```python
from build123d import *

# Parameters (mm, degrees)
BOSS_EXTRUDE1_DEPTH = 7.5
SKETCH3_W           = 56.5
SKETCH3_H           = 84.5
SKETCH3_W_2         = 54.5
SKETCH3_H_2         = 69.44
CUT_EXTRUDE1_DEPTH  = 5
SKETCH4_W           = 54.5
SKETCH4_H           = 9.636528607
CUT_EXTRUDE2_DEPTH  = 5
SKETCH5_W           = 32
SKETCH5_H           = 23.1
BOSS_EXTRUDE2_DEPTH = 49
SKETCH6_W           = 32
SKETCH6_H           = 23.1
BOSS_EXTRUDE3_DEPTH = 49
SKETCH7_R           = 5.000174567
BOSS_EXTRUDE4_DEPTH = 20


with BuildPart() as part:
    # Sketch2 → Boss-Extrude1 (new body)
    with BuildSketch(Plane.XY):
        with BuildLine():
            Line((-82.896774194, 76.290322581), (37.103225806, 76.290322581))
            ThreePointArc((37.103225806, 76.290322581), (44.174293618, 73.361390393), (47.103225806, 66.290322581))
            Line((47.103225806, 66.290322581), (47.103225806, -88.709677419))
            ThreePointArc((47.103225806, -88.709677419), (44.174293618, -95.780745231), (37.103225806, -98.709677419))
            Line((37.103225806, -98.709677419), (-82.896774194, -98.709677419))
            ThreePointArc((-82.896774194, -98.709677419), (-89.967842005, -95.780745231), (-92.896774194, -88.709677419))
            Line((-92.896774194, -88.709677419), (-92.896774194, 66.290322581))
            ThreePointArc((-92.896774194, 66.290322581), (-89.967842005, 73.361390393), (-82.896774194, 76.290322581))
        make_face()
    extrude(amount=BOSS_EXTRUDE1_DEPTH)

    # Sketch3 → Cut-Extrude1 (cut)
    with BuildSketch(Plane.XY.offset(7.5)):
        with Locations((-44.646774194, 27.040322581)):
            Rectangle(SKETCH3_W, SKETCH3_H)
        with Locations((-44.646774194, -56.989677419)):
            Rectangle(SKETCH3_W_2, SKETCH3_H_2)
    extrude(amount=-CUT_EXTRUDE1_DEPTH, mode=Mode.SUBTRACT)

    # Sketch4 → Cut-Extrude2 (cut)
    with BuildSketch(Plane.XY.offset(7.5)):
        with Locations((-44.646774194, -96.527941723)):
            Rectangle(SKETCH4_W, SKETCH4_H)
    extrude(amount=-CUT_EXTRUDE2_DEPTH, mode=Mode.SUBTRACT)

    # Sketch5 → Boss-Extrude2 (add)
    with BuildSketch(Plane.XY.offset(7.5)):
        with Locations((4.603225806, 57.39165706)):
            Rectangle(SKETCH5_W, SKETCH5_H)
        with BuildLine():
            Line((-6.396774194, 65.94165706), (15.603225806, 65.94165706))
            ThreePointArc((15.603225806, 65.94165706), (17.017439369, 65.355870623), (17.603225806, 63.94165706))
            Line((17.603225806, 63.94165706), (17.603225806, 50.84165706))
            ThreePointArc((17.603225806, 50.84165706), (17.017439369, 49.427443498), (15.603225806, 48.84165706))
            Line((15.603225806, 48.84165706), (-6.396774194, 48.84165706))
            ThreePointArc((-6.396774194, 48.84165706), (-7.810987756, 49.427443498), (-8.396774194, 50.84165706))
            Line((-8.396774194, 50.84165706), (-8.396774194, 63.94165706))
            ThreePointArc((-8.396774194, 63.94165706), (-7.810987756, 65.355870623), (-6.396774194, 65.94165706))
        make_face(mode=Mode.SUBTRACT)
    extrude(amount=BOSS_EXTRUDE2_DEPTH)

    # Sketch6 → Boss-Extrude3 (add)
    with BuildSketch(Plane.XY.offset(7.5)):
        with Locations((4.603225806, -79.809677419)):
            Rectangle(SKETCH6_W, SKETCH6_H)
        with BuildLine():
            Line((-6.396774194, -71.259677419), (15.603225806, -71.259677419))
            ThreePointArc((15.603225806, -71.259677419), (17.017439369, -71.845463857), (17.603225806, -73.259677419))
            Line((17.603225806, -73.259677419), (17.603225806, -86.359677419))
            ThreePointArc((17.603225806, -86.359677419), (17.017439369, -87.773890982), (15.603225806, -88.359677419))
            Line((15.603225806, -88.359677419), (-6.396774194, -88.359677419))
            ThreePointArc((-6.396774194, -88.359677419), (-7.810987756, -87.773890982), (-8.396774194, -86.359677419))
            Line((-8.396774194, -86.359677419), (-8.396774194, -73.259677419))
            ThreePointArc((-8.396774194, -73.259677419), (-7.810987756, -71.845463857), (-6.396774194, -71.259677419))
        make_face(mode=Mode.SUBTRACT)
    extrude(amount=BOSS_EXTRUDE3_DEPTH)

    # Sketch7 → Boss-Extrude4 (add)
    with BuildSketch(Plane.XY.offset(7.5)):
        with Locations(Location((-82.896774194, 66.290322581, 0), (0, 0, 180))):
            Circle(SKETCH7_R)
        with Locations(Location((37.103225806, 66.290322581, 0), (0, 0, 180))):
            Circle(SKETCH7_R)
        with Locations(Location((-82.896774194, -88.709677419, 0), (0, 0, 180))):
            Circle(SKETCH7_R)
        with Locations(Location((37.103225806, -88.709677419, 0), (0, 0, 180))):
            Circle(SKETCH7_R)
    extrude(amount=BOSS_EXTRUDE4_DEPTH)


solid = part.part
```
Verification items for the finished model (mm, model axes). A direction names the side the tool comes from. Round coordinates to 2 decimals unless told otherwise and drop trailing zeros. Write each loop counter-clockwise with the first axis right and the second up, starting at its lowest first coordinate (ties: lowest second). Pieces come first, ordered by that corner, then holes. Notation, with made-up numbers: (-12.75, 24) -> (41.25, 24) arc R19 ccw to (41.25, 45) -> close; hole circle Ø4 at (5, 1.25). An arc over 180 degrees is marked (long way). Write each question's results on one line, items separated by ' | '. Start each with the question number.
1. Draft check along Y on faces 1 (the flat face through (-9, -98.71, 3)), 2 (the flat face through (37, -89, 27.5)), 3 (the flat face through (-45, -15.21, 5)). Enter one of: +Y half, -Y half, draft (parallel to the pull), parting line (faces both ways), or undercut.
2. Cross-section at A-A (z = 24). Enter the section's corners in (x, y), then the cut area to 3 significant figures.
3. Set-up check for faces 4 (the cylindrical face through (44.252, -95.703, 3.698)), 5 (the flat face through (-16.397, 26, 5)), 6 (the flat face through (37, 66, 27.5)), 7 (the flat face through (-71.897, -61, 5)), 8 (the flat face through (-83, 66, 27.5)): record each of +Z, -Z, +X, -X, +Y, -Y from which the full face is reachable in a straight line by a thin tool's end or side.
4. Cross-section at B-B (z = 50.5). Enter the section's corners in (x, y).
5. Cross-section at D-D (y = -52). Enter the section's corners in (x, z), then the cut area to 4 significant figures.
6. Depth check by flat-ended pin: P1, Ø2.5, axis at x = -43, z = 6, coming from the -Y side; P2, Ø8, axis at y = -75, z = 33, coming from the +X side; P3, Ø6, axis at x = 16.5, z = 36.5, coming from the -Y side; P4, Ø1.5, axis at y = 44, z = 22.5, coming from the -X side. Enter the tip coordinate at first touch or a pass-through.
7. Cross-section at C-C (x = -47.5). Enter the section's corners in (y, z).
8. Material ranges on probe 1 along Y at (x, z) = (2.5, 33.5); probe 2 along X at (y, z) = (57, 43.5); probe 3 along Z at (x, y) = (-57, 1.5), recorded low to high. Write a range as from..to.
Solutions:
1) face 1: -Y half | face 2: draft | face 3: undercut
2) outline: circle Ø10 at (-82.9, -88.71); circle Ø10 at (-82.9, 66.29); (-11.4, -91.36) -> (20.6, -91.36) -> (20.6, -68.26) -> (-11.4, -68.26) -> close; (-11.4, 45.84) -> (20.6, 45.84) -> (20.6, 68.94) -> (-11.4, 68.94) -> close; circle Ø10 at (37.1, -88.71); circle Ø10 at (37.1, 66.29); hole (-8.4, -86.36) arc R2 ccw to (-6.4, -88.36) -> (15.6, -88.36) arc R2 ccw to (17.6, -86.36) -> (17.6, -73.26) arc R2 ccw to (15.6, -71.26) -> (-6.4, -71.26) arc R2 ccw to (-8.4, -73.26) -> close; hole (-8.4, 50.84) arc R2 ccw to (-6.4, 48.84) -> (15.6, 48.84) arc R2 ccw to (17.6, 50.84) -> (17.6, 63.94) arc R2 ccw to (15.6, 65.94) -> (-6.4, 65.94) arc R2 ccw to (-8.4, 63.94) -> close | area: 910 mm2
3) face 4: +Z, -Z, +X, -Y | face 5: +Z | face 6: +Z, +X, +Y, -Y | face 7: +Z, -Y | face 8: +Z, -X, +Y, -Y
4) outline: (-11.4, -91.36) -> (20.6, -91.36) -> (20.6, -68.26) -> (-11.4, -68.26) -> close; (-11.4, 45.84) -> (20.6, 45.84) -> (20.6, 68.94) -> (-11.4, 68.94) -> close; hole (-8.4, -86.36) arc R2 ccw to (-6.4, -88.36) -> (15.6, -88.36) arc R2 ccw to (17.6, -86.36) -> (17.6, -73.26) arc R2 ccw to (15.6, -71.26) -> (-6.4, -71.26) arc R2 ccw to (-8.4, -73.26) -> close; hole (-8.4, 50.84) arc R2 ccw to (-6.4, 48.84) -> (15.6, 48.84) arc R2 ccw to (17.6, 50.84) -> (17.6, 63.94) arc R2 ccw to (15.6, 65.94) -> (-6.4, 65.94) arc R2 ccw to (-8.4, 63.94) -> close
5) outline: (-92.9, 0) -> (47.1, 0) -> (47.1, 7.5) -> (-17.4, 7.5) -> (-17.4, 2.5) -> (-71.9, 2.5) -> (-71.9, 7.5) -> (-92.9, 7.5) -> close | area: 777.5 mm2
6) P1: stops at y = -22.27 | P2: stops at x = 20.6 | P3: stops at y = -91.36 | P4: passes through
7) outline: (-98.71, 0) -> (76.29, 0) -> (76.29, 7.5) -> (69.29, 7.5) -> (69.29, 2.5) -> (-15.21, 2.5) -> (-15.21, 7.5) -> (-22.27, 7.5) -> (-22.27, 2.5) -> (-98.71, 2.5) -> close
8) probe 1: y = -91.36..-88.36, -71.26..-68.26, 45.84..48.84, 65.94..68.94 | probe 2: x = -11.4..-8.4, 17.6..20.6 | probe 3: z = 0..2.5
